Build history of the part. All positions in model axes, mm. Face numbers are marked on the shaded views. A direction names the side the tool comes from. Give positions to 0.01 mm unless a question says otherwise; leave off trailing zeros. Order: outer loops, then holes, each group sorted by start corner. A loop starts at its lowest first (then second) coordinate and runs counter-clockwise, first axis right, second up. Notation, with made-up numbers: M -30.75,8 L -8.75,8 A6 cw -8.75,13 Z; hole C 89,-31.75 d1. An arc over 180 degrees is marked long. Use CSV: the item, a comma, the result in double quotes. Start each with the question number.
Item 1: Pin check, flat tips, straight feed: P1, Ø8, axis at x = -40, y = -62.5, coming from the -Z side; P2, Ø1.5, axis at x = -54, y = -51, coming from the +Z side; P3, Ø3, axis at x = -7.5, y = 52.5, coming from the +Z side. Stop position of each tip, or through.
Item 2: Wall check: line 1 along Z through (x, y) = (-30, 4); line 2 along X through (y, z) = (-2.5, 142.5); line 3 along Z through (x, y) = (-6.5, 45). Give the ranges that are in metal, low to high.
Item 3: Which spindle directions (+Z, -Z, +X, -X, +Y, -Y) get a long thin tool onto all of the face, cutting with end or side? Do the marked faces 1 and 2. Say none if no direction does.
Item 4: Band-saw the part on A-A on z = 170.5. Write the cut outline in (x, y).
from build123d import *

# Parameters (mm, degrees)
F2_R     = 25
F3_DEPTH = 260
F4_R     = 5
F5_R     = 5


with BuildPart() as f1:
    # F0 (on Front) → F1 (revolve)
    with BuildSketch(Plane.XZ):
        with BuildLine():
            ThreePointArc((0, -80), (56.568542, -56.568542), (80, 0))
            ThreePointArc((80, 0), (56.568542, 56.568542), (0, 80))
            Line((0, 80), (0, -80))
        make_face()
    revolve(axis=Axis((0, 0, 0), (0, 0, -1)))

    # F2 (on Top) → F3 (join)
    with BuildSketch(Plane.XY):
        Circle(F2_R)
    extrude(amount=F3_DEPTH)

    # F4
    f4_edges = [f1.edges().sort_by_distance(p)[0] for p in [
        (-25, 0, 260),
    ]]
    fillet(f4_edges, radius=F4_R)

    # F5
    f5_edges = [f1.edges().sort_by_distance(p)[0] for p in [
        (-25, 0, 75.993421),
    ]]
    fillet(f5_edges, radius=F5_R)


solid = f1.part
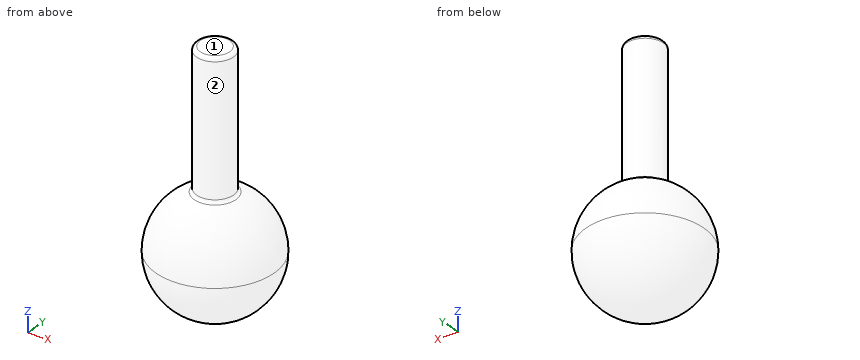
Model answer:
1,P1,"stops at z = -38.36"
1,P2,"stops at z = 31.53"
1,P3,"stops at z = 61.19"
2,line 1,"z = -74.05 to 74.05"
2,line 2,"x = -24.87 to 24.87"
2,line 3,"z = -65.82 to 65.82"
3,face 1,"+Z, +X, -X, +Y, -Y"
3,face 2,"+Z"
4,outline,"C 0,0 d50"
